Autodesk Inventor part; units mm, degrees
ref_plane "YZ Plane" through (0, 0, 0) normal (1, 0, 0) x (0, 1, 0)
ref_plane "XZ Plane" through (0, 0, 0) normal (0, 1, 0) x (-1, 0, 0)
ref_plane "XY Plane" through (0, 0, 0) normal (0, 0, 1) x (1, 0, 0)
sketch "Sketch1" plane through (0, 0, 0) normal (0, 1, 0) x (-1, 0, 0)
  line L0 (23.75, 26) -> (-23.75, 26)
  line L1 (-23.75, 26) -> (-23.75, -26)
  line L2 (-23.75, -26) -> (23.75, -26)
  line L3 (23.75, -26) -> (23.75, 26)
  line L4 (23.75, 26) -> (-23.75, -26) construction
  line L5 (-23.75, 26) -> (23.75, -26) construction
  point P0 (0, 0)
  point P1 (0, -26)
  dimension "d0" = 47.5
  dimension "d1" = 52
extrude "Extrusion1" add sketch "Sketch1" along normal blind 3
fillet "Fillet1" radius 3 4 edges at (0, 3, -26) (-23.75, 3, 0) (0, 3, 26) (23.75, 3, 0)
sketch "Sketch2" plane through (0, 0, 0) normal (0, -1, 0) x (1, 0, 0)
  line L0 (-23.75, -26) -> (-23.75, 26) construction
  line L1 (23.75, -26) -> (-23.75, -26) construction
  line L2 (21, 23.25) -> (-21, 23.25)
  line L3 (-21, 23.25) -> (-21, -23.25)
  line L4 (-21, -23.25) -> (21, -23.25)
  line L5 (21, -23.25) -> (21, 23.25)
  line L6 (21, 23.25) -> (-21, -23.25) construction
  line L7 (-21, 23.25) -> (21, -23.25) construction
  line L8 (16.5, -23.25) -> (9.5, -23.25)
  line L9 (9.5, -23.25) -> (9.5, -21.75)
  line L10 (9.5, -21.75) -> (16.5, -21.75)
  line L11 (16.5, -21.75) -> (16.5, -23.25)
  point P0 (0, 0)
  dimension "d5" = 2.75
  dimension "d6" = 2.75
  dimension "d7" = 7
  dimension "d8" = 1.5
  dimension "d9" = 9.5
extrude "Extrusion2" add sketch "Sketch2" along normal blind 4 contours L4 L9 L10 L11
sketch "Sketch3" plane through (16.5, 0, -23.25) normal (0, 0, -1) x (-1, 0, 0)
  line L0 (7, 0) -> (7, -4) construction
  line L1 (0, -4) -> (7, -4)
  line L2 (7, -4) -> (7, -2.5)
  line L3 (7, -2.5) -> (0, -2.5)
  line L4 (0, -2.5) -> (0, -4)
  point P0 (16.5, 0)
  dimension "d12" = 1.5
extrude "Extrusion3" add sketch "Sketch3" along normal blind 0.8
chamfer "Chamfer1" distance 0.8 angle 45 1 edges at (13, -4, -24.05)
fillet "Fillet2" radius 3 4 edges at (22.8713, 2.1213, 25.1213) (-22.8713, 2.1213, 25.1213) (-22.8713, 2.1213, -25.1213) (22.8713, 2.1213, -25.1213)
mirror "Mirror1" about plane through (0, 0, 0) normal (1, 0, 0) of "Extrusion2", "Chamfer1", "Extrusion3"
mirror "Mirror2" about plane through (0, 0, 0) normal (0, 0, 1) of "Extrusion2", "Chamfer1", "Extrusion3", "Mirror1"
properties part number "capac baterie"
Check sheet for the modelled part. Datum: model origin and axes. Units: mm. A direction names the side the tool comes from. Coordinates: 2 decimals unless noted, no trailing zeros. Order: outer loops, then holes, each group sorted by start corner. A loop starts at its lowest first (then second) coordinate and runs counter-clockwise, first axis right, second up. Notation, with made-up numbers: M -40,69 L -4,69 A34 cw -4,99 Z; hole C 57,-4 d9. An arc over 180 degrees is marked long. Write each question's results on one line, items separated by ' | '. Start each with the question number.
1. Material ranges on probe 1 along Z at (x, y) = (-12, -3); probe 2 along Y at (x, z) = (-17, -5); probe 3 along Z at (x, y) = (-15.5, -0.5), recorded low to high.
2. Mould release check, pull along Z, two halves, no side actions. Record for faces 6 (the face through (13, -1, -23.25)), 7 (the face through (-13, -2, 21.75)), 8 (the face through (16.5, -2, -23)): +Z half, -Z half, draft (parallel to the pull), parting line (faces both ways), or undercut.
3. Go/stop test with flat-tipped pins: P1, Ø0.8, axis at x = 12.5, y = -2, coming from the +Z side; P2, Ø2.5, axis at y = -2.5, z = 22.5, coming from the +X side; P3, Ø0.8, axis at x = 13.5, y = -3, coming from the +Z side. Record where each tip stops, or that it passes through.
4. Access from +Z, -Z, +X, -X, +Y, -Y to the whole of each face (thin tool, end or side, straight path). Record for faces 1 (the face through (-13, -2, -21.75)), 2 (the face through (-9.5, -2, -23)), 3 (the face through (16.5, -2, 23)), 4 (the face through (13, -1, 23.25)), 5 (the face through (-16.5, -2, 23)).
5. Cross-section at A-A on y = -1.75. Record the cut outline in (x, z), and give its area (3 significant figures).
Checks:
1) probe 1: z = -24.05 to -21.75, 21.75 to 24.05 | probe 2: y = 0 to 3 | probe 3: z = -23.25 to -21.75, 21.75 to 23.25
2) face 6: -Z half | face 7: undercut | face 8: draft
3) P1: stops at z = 23.25 | P2: stops at x = 16.5 | P3: stops at z = 24.05
4) face 1: +X, -X, -Y | face 2: +Z, -Z, -Y | face 3: +Z, -Z, +X, -Y | face 4: +Z, +X, -X | face 5: +Z, -Z, -X, -Y
5) outline: M -16.5,-23.25 L -9.5,-23.25 L -9.5,-21.75 L -16.5,-21.75 Z; M -16.5,21.75 L -9.5,21.75 L -9.5,23.25 L -16.5,23.25 Z; M 9.5,-23.25 L 16.5,-23.25 L 16.5,-21.75 L 9.5,-21.75 Z; M 9.5,21.75 L 16.5,21.75 L 16.5,23.25 L 9.5,23.25 Z | area: 42.0 mm²
